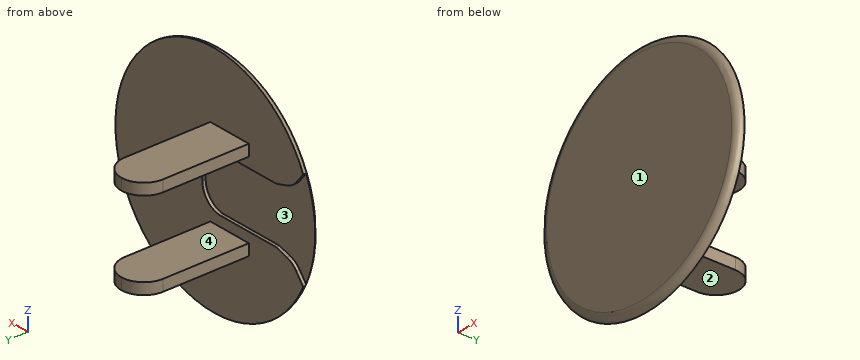
Autodesk Inventor part; units mm, degrees
ref_plane "YZ Plane" through (0, 0, 0) normal (1, 0, 0) x (0, 1, 0)
ref_plane "XZ Plane" through (0, 0, 0) normal (0, 1, 0) x (-1, 0, 0)
ref_plane "XY Plane" through (0, 0, 0) normal (0, 0, 1) x (1, 0, 0)
sketch "Sketch1" plane through (0, 0, 0) normal (0, 1, 0) x (-1, 0, 0)
  circle A0 centre (0, 0) radius 16.9164
  dimension "d0" = 33.8328
extrude "Extrusion1" add sketch "Sketch1" along normal blind 1
fillet "Fillet1" radius 1.016 1 edges at (16.9164, 0, 0)
sketch "Sketch2" plane through (0, 1, 0) normal (0, 1, 0) x (1, 0, 0)
  circle A0 centre (0, 0) radius 16.9164
  line L0 (-0.1238, 7.1755) -> (0.6262, 7.1755) construction
  line L1 (-0.1238, 7.1755) -> (-0.8738, 7.1755) construction
  line L2 (0.6262, 7.1755) -> (-5.9778, 7.1755) construction
  line L3 (-5.9778, 7.1755) -> (-5.9778, 5.5245)
  line L4 (-5.9778, 5.5245) -> (0.6262, 5.5245)
  line L5 (0.6262, 5.5245) -> (0.6262, 7.1755)
  line L6 (0.6262, -7.1755) -> (-5.9778, -7.1755)
  line L7 (-5.9778, -7.1755) -> (-5.9778, -5.5245)
  line L8 (-5.9778, -5.5245) -> (0.6262, -5.5245)
  line L9 (0.6262, -5.5245) -> (0.6262, -7.1755)
  line L10 (0.6262, 6.35) -> (-5.9778, 6.35) construction
  line L11 (0.6262, -6.35) -> (-5.9778, -6.35) construction
  line L12 (-5.9778, 7.1755) -> (0.6262, 7.1755)
  line L13 (-2.6758, 6.35) -> (-2.6758, 16.7034) construction
  line L14 (-2.6758, -6.35) -> (-2.6758, -16.7034) construction
  line L15 (-5.9778, 7.1755) -> (-15.3192, 7.1755) construction
  line L16 (-5.9778, -7.1755) -> (-15.3192, -7.1755) construction
  line L17 (-15.3192, 7.1755) -> (-14.0913, 5.6461)
  line L18 (-12.4965, 4.5835) -> (-10.6485, 4.0497)
  line L19 (-10.6485, 4.0497) -> (-1.1572, 4.0497)
  line L20 (-10.6485, 4.0497) -> (-13.4621, 4.8624) construction
  line L21 (-13.4621, 4.8624) -> (-15.3192, 7.1755) construction
  line L22 (2.0178, 0.8747) -> (2.0178, 0)
  line L23 (2.0178, 0) -> (-20.8537, 0) construction
  line L24 (-15.3192, -7.1755) -> (-14.0913, -5.6461)
  line L25 (-12.4965, -4.5835) -> (-10.6485, -4.0497)
  line L26 (-10.6485, -4.0497) -> (-1.1572, -4.0497)
  line L27 (-10.6485, -4.0497) -> (-13.4621, -4.8624) construction
  line L28 (2.0178, -0.8747) -> (2.0178, 0)
  arc A1 (2.0178, 0.8747) -> (-1.1572, 4.0497) centre (-1.1572, 0.8747) ccw
  arc A2 (-1.1572, -4.0497) -> (2.0178, -0.8747) centre (-1.1572, -0.8747) ccw
  arc A3 (-14.0913, 5.6461) -> (-12.4965, 4.5835) centre (-11.6155, 7.6338) ccw
  arc A4 (-12.4965, -4.5835) -> (-14.0913, -5.6461) centre (-11.6155, -7.6338) ccw
  point P0 (-0.1238, -4.822)
  point P1 (-13.4621, 4.8624)
  point P2 (2.0178, 4.0497)
  point P3 (-13.4621, -4.8624)
  point P4 (2.0178, -4.0497)
  dimension "d17" = 6.604
  dimension "d18" = 1.651
  dimension "d20" = 12.7
  dimension "d21" = 6.604
  dimension "d22" = 1.651
  dimension "d28" = 3.175
sketch "Sketch3" plane through (0, 1, 0) normal (0, 1, 0) x (1, 0, 0)
  point P0 (0, 0)
extrude "Extrusion2" add sketch "Sketch2" along normal blind 15.9 contours L6 L7 L8 L9
extrude "Extrusion3" add sketch "Sketch2" along normal blind 15.9 contours L12 L5 L4 L3
fillet "Fillet2" radius 3.302 4 edges at (-5.9778, 16.9, 6.35) (0.6262, 16.9, 6.35) (-5.9778, 16.9, -6.35) (0.6262, 16.9, -6.35)
extrude "Extrusion4" cut sketch "Sketch2" against normal blind 0.5 contours L17 A3 L18 L19 A1 L22 L28 A2 L26 L25 A4 L24 A0 picked at (-4.321, -1.3499)
properties part number "Replacemnet part(wall socket)"
Geometry: final body of the model. Coordinates: model frame, mm. Face numbers are marked on the shaded views. Coordinates: 2 decimals unless noted, no trailing zeros. Order: outer loops, then holes, each group sorted by start corner. A loop starts at its lowest first (then second) coordinate and runs counter-clockwise, first axis right, second up. Notation, with made-up numbers: (66, 35) -> (111, 35) arc R20 ccw to (111, 52) -> close; hole circle Ø11 at (22.5, -30). An arc over 180 degrees is marked (long way). Write each question's results on one line, items separated by ' | '. Start each with the question number.
1) Mould query, pull axis Z, two halves, no side actions, for the marked faces 1, 2, 3 and 4. Classes: released by +Z, released by -Z, zero draft, split by the parting line, or undercut.
2) Cut plane A-A, the plane y = 10. Output: boundary loops of the cut face in (x, z), and give its area (3 significant figures).
3) First-contact query: pin 1 (0.6 mm diameter, centred on x = -5, y = 0.5, fed in from -Z); pin 2 (4 mm diameter, centred on x = -3, y = 11, fed in from -Z); pin 3 (3 mm diameter, centred on x = 9, z = 5.5, fed in from +Y). Flat tips, straight axial feed; report the tip coordinate or a pass-through.
4) Material intervals for line 1 along X through (y, z) = (11.75, -7); line 2 along Z through (x, y) = (-4, 12); line 3 along Y through (x, z) = (7, -11.5), sorted ascending.
Checks:
1) face 1: zero draft | face 2: released by -Z | face 3: undercut | face 4: undercut
2) outline: (-5.98, -7.18) -> (0.63, -7.18) -> (0.63, -5.52) -> (-5.98, -5.52) -> close; (-5.98, 5.52) -> (0.63, 5.52) -> (0.63, 7.18) -> (-5.98, 7.18) -> close | area: 21.8 mm^2
3) pin 1: z = -16.18 | pin 2: z = -7.18 | pin 3: y = 1
4) line 1: -5.98 to 0.63 | line 2: -7.18 to -5.52, 5.52 to 7.18 | line 3: 0 to 1
